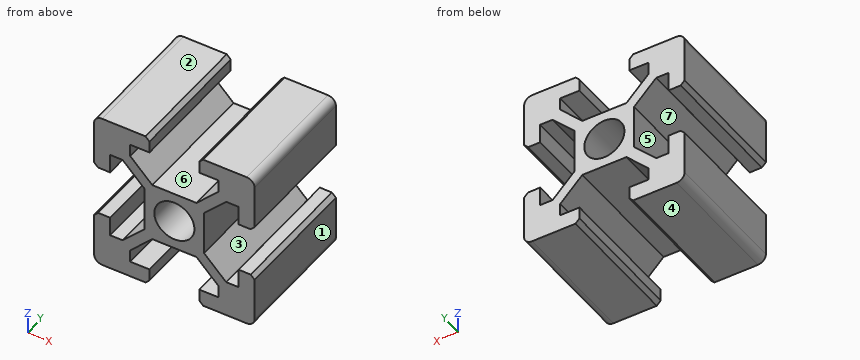
```python
from build123d import *

# Parameters (mm, degrees)
SKETCH1_R           = 2.5
BOSS_EXTRUDE1_DEPTH = 16


with BuildPart() as part:
    # Sketch1 → Boss-Extrude1 (new body)
    with BuildSketch(Plane(origin=(0, 0, 0), x_dir=(1, 0, 0), z_dir=(0, 1, 0))):
        with BuildLine():
            Line((3.6, 10), (9, 10))
            ThreePointArc((9, 10), (9.707106781, 9.707106781), (10, 9))
            Line((10, 9), (10, 3.6))
            Line((10, 3.6), (9.5, 3.1))
            Line((9.5, 3.1), (8, 3.1))
            Line((8, 3.1), (8, 5.5))
            Line((8, 5.5), (6.45, 5.5))
            Line((6.45, 5.5), (3.7, 2.75))
            Line((3.7, 2.75), (3.7, -2.75))
            Line((3.7, -2.75), (6.45, -5.5))
            Line((6.45, -5.5), (8, -5.5))
            Line((8, -5.5), (8, -3.1))
            Line((8, -3.1), (9.5, -3.1))
            Line((9.5, -3.1), (10, -3.6))
            Line((10, -3.6), (10, -9))
            ThreePointArc((10, -9), (9.707106781, -9.707106781), (9, -10))
            Line((9, -10), (3.6, -10))
            Line((3.6, -10), (3.1, -9.5))
            Line((3.1, -9.5), (3.1, -8))
            Line((3.1, -8), (5.5, -8))
            Line((5.5, -8), (5.5, -6.45))
            Line((5.5, -6.45), (2.75, -3.7))
            Line((2.75, -3.7), (-2.75, -3.7))
            Line((-2.75, -3.7), (-5.5, -6.45))
            Line((-5.5, -6.45), (-5.5, -8))
            Line((-5.5, -8), (-3.1, -8))
            Line((-3.1, -8), (-3.1, -9.5))
            Line((-3.1, -9.5), (-3.6, -10))
            Line((-3.6, -10), (-9, -10))
            ThreePointArc((-9, -10), (-9.707106781, -9.707106781), (-10, -9))
            Line((-10, -9), (-10, -3.6))
            Line((-10, -3.6), (-9.5, -3.1))
            Line((-9.5, -3.1), (-8, -3.1))
            Line((-8, -3.1), (-8, -5.5))
            Line((-8, -5.5), (-6.45, -5.5))
            Line((-6.45, -5.5), (-3.7, -2.75))
            Line((-3.7, -2.75), (-3.7, 2.75))
            Line((-3.7, 2.75), (-6.45, 5.5))
            Line((-6.45, 5.5), (-8, 5.5))
            Line((-8, 5.5), (-8, 3.1))
            Line((-8, 3.1), (-9.5, 3.1))
            Line((-9.5, 3.1), (-10, 3.6))
            Line((-10, 3.6), (-10, 9))
            ThreePointArc((-10, 9), (-9.707106781, 9.707106781), (-9, 10))
            Line((-9, 10), (-3.6, 10))
            Line((-3.6, 10), (-3.1, 9.5))
            Line((-3.1, 9.5), (-3.1, 8))
            Line((-3.1, 8), (-5.5, 8))
            Line((-5.5, 8), (-5.5, 6.45))
            Line((-5.5, 6.45), (-2.75, 3.7))
            Line((-2.75, 3.7), (2.75, 3.7))
            Line((2.75, 3.7), (5.5, 6.45))
            Line((5.5, 6.45), (5.5, 8))
            Line((5.5, 8), (3.1, 8))
            Line((3.1, 8), (3.1, 9.5))
            Line((3.1, 9.5), (3.6, 10))
        make_face()
        with Locations(Location((0, 0, 0), (0, 0, 270))):
            Circle(SKETCH1_R, mode=Mode.SUBTRACT)
    extrude(amount=BOSS_EXTRUDE1_DEPTH)


solid = part.part
```
Work out the finished part from the listing and answer in its coordinate system (mm). Face numbers are marked on the shaded views. A direction names the side the tool comes from. Round coordinates to 2 decimals unless told otherwise and drop trailing zeros. Write each loop counter-clockwise with the first axis right and the second up, starting at its lowest first coordinate (ties: lowest second). Pieces come first, ordered by that corner, then holes. Notation, with made-up numbers: (12, -37) - (32, -37) arc R26 cw to (32, -2) - close; hole circle Ø6 at (-23.75, 31.25). An arc over 180 degrees is marked (long way). Return JSON: item names as keys, results as strings. Group by question number.
Q1. Find the intervals of material crossed by L1, parallel to X at y = 7.25, z = 0; L2, parallel to Z at x = -8.75, y = 6.5; L3, parallel to X at y = 5, z = -3.75, in increasing order.
Q2. For the marked faces 5, 6 and 7, determine the directions among +Z, -Z, +X, -X, +Y, -Y from which every point of the face is accessible in a straight line to the end or side of a thin tool.
Q3. The part is cut by section B-B on z = 0. Write down the section's boundary in (x, y).
Q4. The part is cut by section A-A on x = 0. Write down the section's boundary in (y, z).
Q5. The mould has two halves that part along Z. Classify the marked faces 1, 2, 3 and 4: released by +Z, released by -Z, zero draft, split by the parting line, or undercut.
Q6. Each of these flat-tipped pins is pushed along its axis until it touches: pin 1 Ø5 at (x, z) = (-2.5, 5) entering from -Y; pin 2 Ø6 at (y, z) = (7.5, -0.5) entering from +X; pin 3 Ø1.6 at (x, y) = (-0.5, 7) entering from -Z; pin 4 Ø4.5 at (x, y) = (1, 4.5) entering from +Z. Where does it stop, or does it pass through?
Solved:
{
 "1": {"L1": "-3.7 to -2.5, 2.5 to 3.7", "L2": "-10 to -3.1, 3.1 to 10", "L3": "-10 to -8, -4.7 to -2.8, 2.8 to 4.7, 8 to 10"},
 "2": {"face 5": "-X, +Y, -Y", "face 6": "+Z, +Y, -Y", "face 7": "+Y, -Y"},
 "3": {"outline": "(-3.7, 0) - (-2.5, 0) - (-2.5, 16) - (-3.7, 16) - close; (2.5, 0) - (3.7, 0) - (3.7, 16) - (2.5, 16) - close"},
 "4": {"outline": "(0, -3.7) - (16, -3.7) - (16, -2.5) - (0, -2.5) - close; (0, 2.5) - (16, 2.5) - (16, 3.7) - (0, 3.7) - close"},
 "5": {"face 1": "zero draft", "face 2": "released by +Z", "face 3": "undercut", "face 4": "released by -Z"},
 "6": {"pin 1": "y = 0", "pin 2": "x = 9.9", "pin 3": "z = -3.7", "pin 4": "z = 9.65"}
}
